CAD build for the part. Positions are in the model's coordinates, mm. Round coordinates to 2 decimals unless told otherwise and drop trailing zeros. Order: outer loops, then holes, each group sorted by start corner. A loop starts at its lowest first (then second) coordinate and runs counter-clockwise, first axis right, second up.
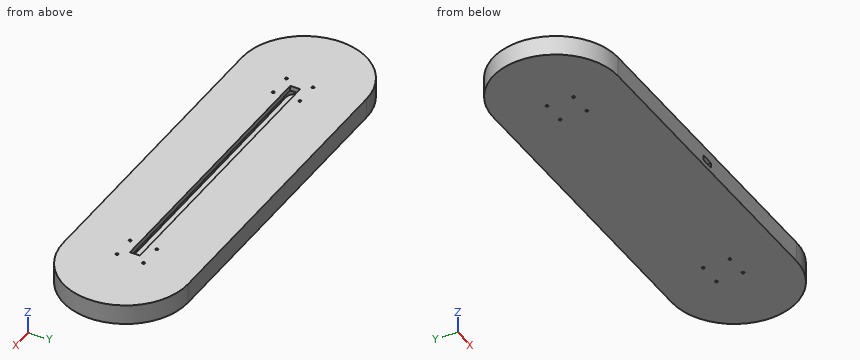
```python
from build123d import *

# Parameters (mm, degrees)
PAD_DEPTH       = 6
POCKET_DEPTH    = 3
SKETCH002_W     = 18.4
SKETCH002_H     = 20.85
POCKET001_DEPTH = 3
SKETCH003_W     = 8
SKETCH003_H     = 1.65
POCKET002_DEPTH = 3
PAD001_DEPTH    = 3
SKETCH005_W     = 170.5
SKETCH005_H     = 5.95
PAD002_DEPTH    = 3
SKETCH007_R     = 0.8
POCKET003_DEPTH = 563.341185


with BuildPart() as part:
    # Sketch → Pad (new body)
    with BuildSketch(Plane.XY):
        with BuildLine():
            ThreePointArc((-95, 37.5), (-132.5, 0), (-95, -37.5))
            Line((-95, -37.5), (95, -37.5))
            ThreePointArc((95, -37.5), (132.5, 0), (95, 37.5))
            Line((-95, 37.5), (95, 37.5))
        make_face()
    extrude(amount=PAD_DEPTH)

    # Sketch001 (on Face6 of Pad) → Pocket (cut)
    with BuildSketch(Plane.XY.offset(6)):
        with BuildLine():
            ThreePointArc((-86, 6), (-92, 0), (-86, -6))
            Line((-86, -6), (86, -6))
            ThreePointArc((86, -6), (92, 0), (86, 6))
            Line((-86, 6), (86, 6))
        make_face()
    extrude(amount=-POCKET_DEPTH, mode=Mode.SUBTRACT)

    # Sketch002 (on Face5 of Pocket) → Pocket001 (cut)
    with BuildSketch(Plane.XY.offset(6)):
        with Locations((0, -25.425)):
            Rectangle(SKETCH002_W, SKETCH002_H)
    extrude(amount=-POCKET001_DEPTH, mode=Mode.SUBTRACT)

    # Sketch003 (on Face5 of Pocket001) → Pocket002 (cut)
    with BuildSketch(Plane.XY.offset(6)):
        with Locations((0, -36.675)):
            Rectangle(SKETCH003_W, SKETCH003_H)
    extrude(amount=-POCKET002_DEPTH, mode=Mode.SUBTRACT)

    # Sketch004 (on Face5 of Pocket002) → Pad001 (join)
    with BuildSketch(Plane.XY.offset(6)):
        with BuildLine():
            ThreePointArc((-95, 37.5), (-132.5, 0), (-95, -37.5))
            Line((-95, -37.5), (95, -37.5))
            ThreePointArc((95, -37.5), (132.5, 0), (95, 37.5))
            Line((-95, 37.5), (95, 37.5))
        make_face()
        with BuildLine():
            ThreePointArc((-86, 6), (-92, 0), (-86, -6))
            Line((-86, -6), (86, -6))
            ThreePointArc((86, -6), (92, 0), (86, 6))
            Line((-86, 6), (86, 6))
        make_face(mode=Mode.SUBTRACT)
    extrude(amount=PAD001_DEPTH)

    # Sketch005 (on Face12 of Pad001) → Pad002 (join)
    with BuildSketch(Plane.XY.offset(9)):
        with BuildLine():
            ThreePointArc((-95, 37.5), (-132.5, 0), (-95, -37.5))
            Line((-95, -37.5), (95, -37.5))
            ThreePointArc((95, -37.5), (132.5, 0), (95, 37.5))
            Line((-95, 37.5), (95, 37.5))
        make_face()
        Rectangle(SKETCH005_W, SKETCH005_H, mode=Mode.SUBTRACT)
    extrude(amount=PAD002_DEPTH)

    # Sketch007 (on Face20 of Pad002) → Pocket003 (cut, through all)
    with BuildSketch(Plane.XY.offset(12)):
        with Locations((-90, -8)):
            Circle(SKETCH007_R)
        with Locations((-90, 8)):
            Circle(SKETCH007_R)
        with Locations((-76, 8)):
            Circle(SKETCH007_R)
        with Locations((-76, -8)):
            Circle(SKETCH007_R)
    pocket003 = extrude(amount=-POCKET003_DEPTH, mode=Mode.SUBTRACT)

    # Mirrored: Pocket003 across Sketch007 V_Axis
    add(pocket003.mirror(Plane(origin=(0, 0, 12), x_dir=(0, 0, 1), z_dir=(1, 0, 0))), mode=Mode.SUBTRACT)


solid = part.part
```
1. Pin check, flat tips, straight feed: P1, Ø2.5, axis at x = 0, z = 5, coming from the -Y side; P2, Ø5, axis at y = 19, z = 9, coming from the -X side; P3, Ø1.5, axis at y = -21, z = 4.5, coming from the -X side; P4, Ø6, axis at y = -19, z = 8.5, coming from the -X side. Stop position of each tip, or through.
2. Drill centre lines: line 1 (Y direction, x = -76, z = 7); line 2 (Y direction, x = -52, z = 8.5); line 3 (Y direction, x = 90, z = 9.5). Where is each one in solid material? Low to high.
3. Cut at D-D, the plane x = -115. Write the cut outline in (y, z).
4. Cut at C-C, the plane x = 31. Write the cut outline in (y, z) (3 decimals).
5. Cut at A-A, the plane y = 0. Write the cut outline in (x, z), and give its area (3 significant figures).
6. Cut at B-B, the plane y = -19.5. Write the cut outline in (x, z).
Outcome:
1. P1: stops at y = -37.5
1. P2: stops at x = -128.67
1. P3: stops at x = -126.56
1. P4: stops at x = -128.92
2. line 1: y = -37.5 to -8.8, -7.2 to -6, 6 to 7.2, 8.8 to 37.5
2. line 2: y = -37.5 to -6, 6 to 37.5
2. line 3: y = -37.5 to -8.8, -7.2 to 7.2, 8.8 to 37.5
3. outline: (-31.72, 0) - (31.72, 0) - (31.72, 12) - (-31.72, 12) - close
4. outline: (-37.5, 0) - (37.5, 0) - (37.5, 12) - (2.975, 12) - (2.975, 9) - (6, 9) - (6, 3) - (-6, 3) - (-6, 9) - (-2.975, 9) - (-2.975, 12) - (-37.5, 12) - close
5. outline: (-132.5, 0) - (132.5, 0) - (132.5, 12) - (85.25, 12) - (85.25, 9) - (92, 9) - (92, 3) - (-92, 3) - (-92, 9) - (-85.25, 9) - (-85.25, 12) - (-132.5, 12) - close
5. area: 1,560 mm2
6. outline: (-127.03, 0) - (127.03, 0) - (127.03, 12) - (-127.03, 12) - close; hole (-9.2, 3) - (9.2, 3) - (9.2, 6) - (-9.2, 6) - close
